```python
from build123d import *

# Parameters (mm, degrees)
CROQUIS1_R              = 3.25
SALIENTE_EXTRUIR1_DEPTH = 3


with BuildPart() as part:
    # Croquis1 → Saliente-Extruir1 (new body)
    with BuildSketch(Plane(origin=(0, 0, 0), x_dir=(1, 0, 0), z_dir=(0, 1, 0))):
        with BuildLine():
            Line((-59, 0), (-17, 0))
            Line((-17, 0), (-17, -9))
            Line((-17, -9), (-14, -9))
            Line((-14, -9), (-14, 0))
            Line((-14, 0), (-5.5, 0))
            ThreePointArc((-5.5, 0), (0, -5.5), (5.5, 0))
            Line((5.5, 0), (14, 0))
            Line((14, 0), (14, -9))
            Line((14, -9), (17, -9))
            Line((17, -9), (17, 0))
            Line((17, 0), (59, 0))
            Line((59, 0), (59, -20))
            Line((59, -20), (62, -20))
            Line((62, -20), (62, 0))
            Line((62, 0), (70, 0))
            ThreePointArc((70, 0), (0, -70), (-70, 0))
            Line((-70, 0), (-62, 0))
            Line((-62, 0), (-62, -20))
            Line((-62, -20), (-59, -20))
            Line((-59, -20), (-59, 0))
        make_face()
        with Locations(Location((0, -50, 0), (0, 0, 270))):
            Circle(CROQUIS1_R, mode=Mode.SUBTRACT)
        with Locations(Location((0, -40, 0), (0, 0, 270))):
            Circle(CROQUIS1_R, mode=Mode.SUBTRACT)
        Polygon((24.748737342, -24.748737342), (19.798989873, -29.69848481), (21.920310217, -31.819805153), (31.819805153, -21.920310217), (29.69848481, -19.798989873), align=None, mode=Mode.SUBTRACT)
        Polygon((-24.748737342, -24.748737342), (-29.69848481, -19.798989873), (-31.819805153, -21.920310217), (-21.920310217, -31.819805153), (-19.798989873, -29.69848481), align=None, mode=Mode.SUBTRACT)
        Polygon((-9, -14), (-9, -17), (9, -17), (9, -14), (0, -14), align=None, mode=Mode.SUBTRACT)
        Polygon((27.577164466, -55.861435714), (55.861435714, -27.577164466), (57.982756057, -29.69848481), (43.840620434, -43.840620434), (29.69848481, -57.982756057), align=None, mode=Mode.SUBTRACT)
        Polygon((-20, -59), (20, -59), (20, -62), (0, -62), (-20, -62), align=None, mode=Mode.SUBTRACT)
        Polygon((-55.861435714, -27.577164466), (-27.577164466, -55.861435714), (-29.69848481, -57.982756057), (-43.840620434, -43.840620434), (-57.982756057, -29.69848481), align=None, mode=Mode.SUBTRACT)
    extrude(amount=SALIENTE_EXTRUIR1_DEPTH)


solid = part.part
```
For this review, take the finished solid that the model builds, in its own axes (mm). A direction names the side the tool comes from. Coordinates: 2 decimals unless noted, no trailing zeros. Write each loop counter-clockwise with the first axis right and the second up, starting at its lowest first coordinate (ties: lowest second). Pieces come first, ordered by that corner, then holes. Notation, with made-up numbers: (-5, 3) -> (12, 3) arc R20 ccw to (12, 31) -> close; hole circle Ø9 at (65.25, 43). An arc over 180 degrees is marked (long way). Put each result on its own line as item: value.
Q1. Wall thickness on L1, parallel to X at y = 0.25, z = 20.5; L2, parallel to X at y = 0.5, z = 47; L3, parallel to X at y = 1.6, z = 40: over which ranges is each line inside the solid? List them lowest first.
From the geometry:
L1: x = -66.93 to -30.4, -29 to 29, 30.4 to 66.93
L2: x = -51.87 to -40.68, -36.44 to -1.25, 1.25 to 36.44, 40.68 to 51.87
L3: x = -57.45 to -47.68, -43.44 to -3.25, 3.25 to 43.44, 47.68 to 57.45
Q2. Take a section at A-A, the plane x = 0. State the section outline as (y, z) points.
From the geometry:
outline: (0, 5.5) -> (3, 5.5) -> (3, 14) -> (0, 14) -> close; (0, 17) -> (3, 17) -> (3, 36.75) -> (0, 36.75) -> close; (0, 43.25) -> (3, 43.25) -> (3, 46.75) -> (0, 46.75) -> close; (0, 53.25) -> (3, 53.25) -> (3, 59) -> (0, 59) -> close; (0, 62) -> (3, 62) -> (3, 70) -> (0, 70) -> close
Q3. Clearance check with flat-ended pins moving along their axes: pin 1 Ø0.9 at (y, z) = (2, 3) entering from +X; pin 2 Ø1.5 at (x, y) = (60, 2) entering from -Z; pin 3 Ø0.9 at (x, y) = (2, 2) entering from -Z. State where each tip first meets the part, or that it passes through.
From the geometry:
pin 1: stops at x = 69.95
pin 2: stops at z = 20
pin 3: stops at z = 4.92
Q4. Take a section at B-B, the plane z = 40. State the section outline as (x, y) points.
From the geometry:
outline: (-57.45, 0) -> (-47.68, 0) -> (-47.68, 3) -> (-57.45, 3) -> close; (-43.44, 0) -> (-3.25, 0) -> (-3.25, 3) -> (-43.44, 3) -> close; (3.25, 0) -> (43.44, 0) -> (43.44, 3) -> (3.25, 3) -> close; (47.68, 0) -> (57.45, 0) -> (57.45, 3) -> (47.68, 3) -> close
Q5. The part is to be moulded in two halves that separate along Z. For faces 4 (the flat face through (59, 1, 10)), 5 (the cylindrical face through (-1.245, 1.479, 43.002)), 6 (the flat face through (-66, 1, 0)), say which applies: +Z half, -Z half, draft (parallel to the pull), parting line (faces both ways), or undercut.
From the geometry:
face 4: draft
face 5: undercut
face 6: -Z half
Q6. Take a section at C-C, the plane x = 52. State the section outline as (y, z) points.
From the geometry:
outline: (0, 0) -> (3, 0) -> (3, 31.44) -> (0, 31.44) -> close; (0, 35.68) -> (3, 35.68) -> (3, 46.86) -> (0, 46.86) -> close
Q7. Take a section at D-D, the plane y = 0.85. Count the separate pieces of the cut face and the enclosed holes in it, then the cut area to 3 significant figures.
From the geometry:
separate pieces: 1
enclosed holes: 8
area: 6,910 mm2
Q8. Tool access review of faces 1 (the flat face through (62, 1, 10)), 2 (the flat face through (1, 3, 35)), 3 (the flat face through (0, 1, 14)): name each direction out of +Z, -Z, +X, -X, +Y, -Y from which nothing blocks a thin tool from reaching the whole face with its end or side.
From the geometry:
face 1: -Z, +Y, -Y
face 2: +Z, -Z, +X, -X, +Y
face 3: +Y, -Y
